Work out the finished part from the listing and answer in its coordinate system (mm). Face numbers are marked on the shaded views. A direction names the side the tool comes from. Coordinates: 2 decimals unless noted, no trailing zeros. Order: outer loops, then holes, each group sorted by start corner. A loop starts at its lowest first (then second) coordinate and runs counter-clockwise, first axis right, second up.
1. The part is cut by section A-A, the plane z = -89. Give the vertices of the cut face in (x, y).
2. A tool of negligible diameter and unlimited length cuts with its end or side. For the marked faces 1 and 2, from which of +Z, -Z, +X, -X, +Y, -Y can it reach the whole face along a straight path? Write none if from no direction.
3. Find the intervals of material crossed by probe 1 along Z at (x, y) = (5.25, -3.75); probe 2 along X at (y, z) = (4.25, -25.5); probe 3 along Y at (x, z) = (-0.75, -117), in increasing order.
4. Flat-ended cylindrical pins translate along their axes: pin 1 Ø2 at (x, z) = (-0.5, -96.5) entering from -Y; pin 2 Ø5 at (x, z) = (6, -121.5) entering from -Y; pin 3 Ø5 at (x, y) = (5.5, -4) entering from -Z; pin 4 Ø1.5 at (x, y) = (-6, -7) entering from -Z. Find the tip coordinate at first contact, or state that the pin passes through.
```python
from build123d import *

# Parameters (mm, degrees)
BOSS_EXTRUDE1_DEPTH = 7.32


with BuildPart() as part:
    # Sketch1 → Boss-Extrude1 (new body)
    with BuildSketch(Plane.XY):
        Polygon((0, 10.779129526), (-9.335, 5.389564763), (-9.335, -5.389564763), (0, -10.779129526), (9.335, -5.389564763), (9.335, 5.389564763), align=None)
    extrude(amount=BOSS_EXTRUDE1_DEPTH)

    # Sketch2 → Revolve1 (revolve)
    with BuildSketch(Plane(origin=(0, 0, 0), x_dir=(0, 0, -1), z_dir=(1, 0, 0))):
        with BuildLine():
            Line((0, 0), (0, 6.6))
            ThreePointArc((0, 6.6), (0.175735931, 6.175735931), (0.6, 6))
            Line((0.6, 6), (159.1, 6))
            Line((159.1, 6), (160, 5.1))
            Line((160, 5.1), (160, 0))
            Line((160, 0), (0, 0))
        make_face()
    revolve(axis=Axis((0, 0, 0), (0, 0, -1)))

    # Sketch3 → Cut-Revolve1 (revolve, cut)
    with BuildSketch(Plane(origin=(0, 0, 0), x_dir=(0, 0, -1), z_dir=(1, 0, 0))):
        Polygon((-7.32, 10.779129526), (-6.48623143, 10.779129526), (-7.32, 9.335), align=None)
        Polygon((-0.15, 10.779129526), (-0.15, 8.78660254), (0, 8.7), (0, 10.779129526), align=None)
    revolve(axis=Axis((0, 0, 12.204941078), (0, 0, -1)), mode=Mode.SUBTRACT)


solid = part.part
```
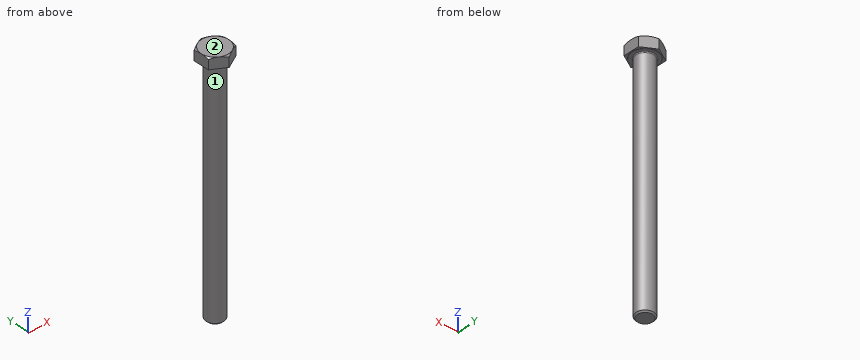
Geometry says:
1. outline: circle Ø12 at (0, 0)
2. face 1: -Z
2. face 2: +Z, +X, -X, +Y, -Y
3. probe 1: z = -0.02 to 7.32
3. probe 2: x = -4.24 to 4.24
3. probe 3: y = -5.95 to 5.95
4. pin 1: stops at y = -6
4. pin 2: stops at y = -4.87
4. pin 3: stops at z = -160
4. pin 4: stops at z = 0
